```python
from build123d import *

# Parameters (mm, degrees)
SCHIZZO1_W                   = 180
SCHIZZO1_H                   = 100
SCHIZZO1_W_2                 = 170
SCHIZZO1_H_2                 = 90
ESTRUSIONE_ESTRUSIONE1_DEPTH = 6
SCHIZZO2_W                   = 0.85
SCHIZZO2_H                   = 100
ESTRUSIONE_ESTRUSIONE2_DEPTH = 170
SCHIZZO3_R                   = 12.5
SCHIZZO3_R_2                 = 9.25
ESTRUSIONE_ESTRUSIONE3_DEPTH = 10
SCHIZZO4_R                   = 5
TAGLIO_ESTRUSIONE1_DEPTH     = 30
SCHIZZO5_W                   = 2
SCHIZZO5_H                   = 50
ESTRUSIONE_ESTRUSIONE4_DEPTH = 2
SCHIZZO10_R                  = 9.25
SCHIZZO10_R_2                = 5
ESTRUSIONE_ESTRUSIONE7_DEPTH = 8.5
SCHIZZO11_R                  = 9.25
SCHIZZO11_R_2                = 5
ESTRUSIONE_ESTRUSIONE8_DEPTH = 8.5
SCHIZZO12_W                  = 27.111147563
SCHIZZO12_H                  = 1.71831217
TAGLIO_ESTRUSIONE2_DEPTH     = 1


with BuildPart() as part:
    # Schizzo1 → Estrusione-Estrusione1 (new body)
    with BuildSketch(Plane.XY):
        Rectangle(SCHIZZO1_W, SCHIZZO1_H)
        Rectangle(SCHIZZO1_W_2, SCHIZZO1_H_2, mode=Mode.SUBTRACT)
    extrude(amount=ESTRUSIONE_ESTRUSIONE1_DEPTH)

    # Schizzo2 → Estrusione-Estrusione2 (add)
    with BuildSketch(Plane(origin=(-85, 0, 0), x_dir=(0, 0, -1), z_dir=(1, 0, 0))):
        with Locations((-5.575, 0)):
            Rectangle(SCHIZZO2_W, SCHIZZO2_H)
    extrude(amount=ESTRUSIONE_ESTRUSIONE2_DEPTH)

    # Schizzo3 → Estrusione-Estrusione3 (add)
    with BuildSketch(Plane(origin=(0, 0, 5.15), x_dir=(-1, 0, 0), z_dir=(0, 0, -1))):
        with Locations((-38, 0.9)):
            Circle(SCHIZZO3_R)
        with Locations((-38, 0.9)):
            Circle(SCHIZZO3_R_2, mode=Mode.SUBTRACT)
        with Locations((38, 1.3)):
            Circle(SCHIZZO3_R)
        with Locations((38, 1.3)):
            Circle(SCHIZZO3_R_2, mode=Mode.SUBTRACT)
    extrude(amount=ESTRUSIONE_ESTRUSIONE3_DEPTH)

    # Schizzo4 → Taglio-Estrusione1 (cut)
    with BuildSketch(Plane(origin=(0, 0, 5.15), x_dir=(-1, 0, 0), z_dir=(0, 0, -1))):
        with Locations((-38, 0.9)):
            Circle(SCHIZZO4_R)
        with Locations((38, 1.3)):
            Circle(SCHIZZO4_R)
    extrude(amount=-TAGLIO_ESTRUSIONE1_DEPTH, mode=Mode.SUBTRACT)

    # Schizzo5 → Estrusione-Estrusione4 (add)
    with BuildSketch(Plane(origin=(0, 0, 0), x_dir=(-1, 0, 0), z_dir=(0, 0, -1))):
        with Locations((-87.5, 0)):
            Rectangle(SCHIZZO5_W, SCHIZZO5_H)
    estrusione_estrusione4 = extrude(amount=ESTRUSIONE_ESTRUSIONE4_DEPTH)

    # Specchia1: Estrusione-Estrusione4 across plane
    add(estrusione_estrusione4.mirror(Plane.ZY))

    # Schizzo10 → Estrusione-Estrusione7 (add)
    with BuildSketch(Plane(origin=(0, 0, 5.15), x_dir=(-1, 0, 0), z_dir=(0, 0, -1))):
        with Locations((-38, 0.9)):
            Circle(SCHIZZO10_R)
        with Locations((-38, 0.9)):
            Circle(SCHIZZO10_R_2, mode=Mode.SUBTRACT)
    extrude(amount=ESTRUSIONE_ESTRUSIONE7_DEPTH)

    # Schizzo11 → Estrusione-Estrusione8 (add)
    with BuildSketch(Plane(origin=(0, 0, 5.15), x_dir=(-1, 0, 0), z_dir=(0, 0, -1))):
        with Locations((38, 1.3)):
            Circle(SCHIZZO11_R)
        with Locations((38, 1.3)):
            Circle(SCHIZZO11_R_2, mode=Mode.SUBTRACT)
    extrude(amount=ESTRUSIONE_ESTRUSIONE8_DEPTH)

    # Schizzo12 → Taglio-Estrusione2 (cut)
    with BuildSketch(Plane(origin=(0, 50, 0), x_dir=(1, 0, 0), z_dir=(0, 1, 0))):
        with Locations((-0.286385361, -2.484235744)):
            Rectangle(SCHIZZO12_W, SCHIZZO12_H)
    extrude(amount=-TAGLIO_ESTRUSIONE2_DEPTH, mode=Mode.SUBTRACT)


solid = part.part
```
Build history of the part. All positions in model axes, mm. A direction names the side the tool comes from. Coordinates: 2 decimals unless noted, no trailing zeros. Order: outer loops, then holes, each group sorted by start corner. A loop starts at its lowest first (then second) coordinate and runs counter-clockwise, first axis right, second up. Notation, with made-up numbers: (72.25, 87) -> (129.25, 87) arc R20 cw to (129.25, 91) -> close; hole circle Ø6 at (75, 33). An arc over 180 degrees is marked (long way). Answer in a Markdown table with one row per item. Add a question column.
Q1. Band-saw the part on C-C, the plane x = -36. List the corners of the cut face in (y, z), then the cut area to 3 significant figures.
Q2. Drop flat-ended pins along their axis: pin 1 (0.6 mm diameter, centred on x = 87.5, z = -1, fed in from +Y); pin 2 (2 mm diameter, centred on x = 87.5, y = -1, fed in from -Z); pin 3 (1.6 mm diameter, centred on y = 9, z = -1, fed in from -X); pin 4 (15 mm diameter, centred on x = -34, y = 5.5, fed in from -Z). Give the stop position or say it passes through.
Q3. Band-saw the part on B-B, the plane y = -41.5. List the corners of the cut face in (x, z), then the cut area to 4 significant figures.
Q4. Band-saw the part on A-A, the plane x = 38. List the corners of the cut face in (y, z).
Q5. Which spindle directions (+Z, -Z, +X, -X, +Y, -Y) get a long thin tool onto all of the face, cutting with end or side? Do faces 4 (the face through (-1, -50, 3)), 5 (the face through (47.92, -6.706, 0.22)). Say none if no direction does.
Q6. Mould opens along X. For faces 1 (the face through (-90, -1, 3)), 2 (the face through (-30.66, -4.33, -4.09)), 3 (the face through (36.2, 10.2, -4.85)) say: +X half, -X half, draft (parallel to the pull), parting line (faces both ways), or undercut.
Q7. Wall check: line 1 along Y through (x, z) = (-38, 3.75); line 2 along X through (y, z) = (-9, 2.5); line 3 along Y through (x, z) = (-75.5, 1.75). Give the ranges that are in metal, low to high. Write a range as [from, to].
Answers follow:
| question | item | result |
|---|---|---|
| 1 | outline | (-50, 0) -> (-45, 0) -> (-45, 5.15) -> (-11.04, 5.15) -> (-11.04, -4.85) -> (-7.73, -4.85) -> (-7.73, -3.35) -> (-3.28, -3.35) -> (-3.28, 6) -> (-50, 6) -> close; (5.88, -3.35) -> (10.33, -3.35) -> (10.33, -4.85) -> (13.64, -4.85) -> (13.64, 5.15) -> (45, 5.15) -> (45, 0) -> (50, 0) -> (50, 6) -> (5.88, 6) -> close |
| 1 | area | 270 mm^2 |
| 2 | pin 1 | y = 25 |
| 2 | pin 2 | z = -2 |
| 2 | pin 3 | x = -88.5 |
| 2 | pin 4 | z = -4.85 |
| 3 | outline | (-90, 0) -> (-85, 0) -> (-85, 5.15) -> (85, 5.15) -> (85, 0) -> (90, 0) -> (90, 6) -> (-90, 6) -> close |
| 3 | area | 204.5 mm^2 |
| 4 | outline | (-50, 0) -> (-45, 0) -> (-45, 5.15) -> (-11.6, 5.15) -> (-11.6, -4.85) -> (-8.35, -4.85) -> (-8.35, -3.35) -> (-4.1, -3.35) -> (-4.1, 6) -> (-50, 6) -> close; (5.9, -3.35) -> (10.15, -3.35) -> (10.15, -4.85) -> (13.4, -4.85) -> (13.4, 5.15) -> (45, 5.15) -> (45, 0) -> (50, 0) -> (50, 6) -> (5.9, 6) -> close |
| 5 | face 4 | +Z, -Z, +X, -X, -Y |
| 5 | face 5 | -Z |
| 6 | face 1 | -X half |
| 6 | face 2 | undercut |
| 6 | face 3 | draft |
| 7 | line 1 | [-50, -45], [-11.2, -3.7], [6.3, 13.8], [45, 50] |
| 7 | line 2 | [-90, -85], [-45.08, -30.92], [30.37, 45.63], [85, 90] |
| 7 | line 3 | [-50, -45], [45, 50] |
